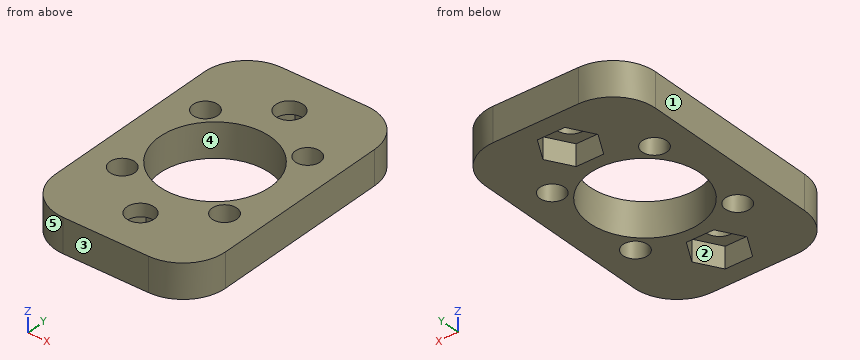
```python
from build123d import *

# Parameters (mm, degrees)
SKETCH_W     = 20
SKETCH_H     = 31.5
SKETCH_R     = 1.6
SKETCH_R_2   = 6.5
SKETCH_R_3   = 1.45
PAD_DEPTH    = 4
POCKET_DEPTH = 2.5
FILLET_R     = 5


with BuildPart() as part:
    # Sketch → Pad (new body)
    with BuildSketch(Plane.XY):
        Rectangle(SKETCH_W, SKETCH_H)
        with Locations((0, 10.75)):
            Circle(SKETCH_R, mode=Mode.SUBTRACT)
        with Locations((0, -10.75)):
            Circle(SKETCH_R, mode=Mode.SUBTRACT)
        Circle(SKETCH_R_2, mode=Mode.SUBTRACT)
        with Locations((6, 6)):
            Circle(SKETCH_R_3, mode=Mode.SUBTRACT)
        with Locations((6, -6)):
            Circle(SKETCH_R_3, mode=Mode.SUBTRACT)
        with Locations((-6, -6)):
            Circle(SKETCH_R_3, mode=Mode.SUBTRACT)
        with Locations((-6, 6)):
            Circle(SKETCH_R_3, mode=Mode.SUBTRACT)
    extrude(amount=PAD_DEPTH)

    # Sketch001 → Pocket (cut)
    with BuildSketch(Plane.XY):
        Polygon((-1.616581, 7.95), (1.616581, 7.95), (3.233162, 10.75), (1.616581, 13.55), (-1.616581, 13.55), (-3.233162, 10.75), align=None)
        Polygon((-1.616581, -7.95), (-3.233162, -10.75), (-1.616581, -13.55), (1.616581, -13.55), (3.233162, -10.75), (1.616581, -7.95), align=None)
    extrude(amount=POCKET_DEPTH, mode=Mode.SUBTRACT)

    # Fillet
    fillet_edges = [part.edges().sort_by_distance(p)[0] for p in [
        (10, -15.75, 2),
        (10, 15.75, 2),
        (-10, 15.75, 2),
        (-10, -15.75, 2),
    ]]
    fillet(fillet_edges, radius=FILLET_R)


solid = part.part
```
Could you check a few things on this model? Use its own coordinates, in mm. Face numbers are marked on the shaded views. A direction names the side the tool comes from. Round coordinates to 2 decimals unless told otherwise and drop trailing zeros. Loops run counter-clockwise (first coordinate to the right, second up) from the corner with the lowest first, then second, coordinate; pieces in that order, holes last. Notation, with made-up numbers: (-35.75, -15) - (21.25, -15) arc R22 cw to (21.25, 9) - close; hole circle Ø7 at (49, 9). An arc over 180 degrees is marked (long way). Answer in a Markdown table with one row per item. Add a question column.
(1) I need wall thicknesses on line 1 along Y through (x, z) = (0, 2.2); line 2 along Y through (x, z) = (0, 3.75); line 3 along X through (y, z) = (-10.75, 3.55). Which ranges of each line are inside material? Lowest first, please.
(2) If we section it at D-D (y = 0): Please give me the cut outline in (x, z).
(3) For the marked faces 1 and 2, which set-ups out of +Z, -Z, +X, -X, +Y, -Y let a thin tool reach every point of the face, with its end or its side?
(4) I'm going to push a flat-ended pin straight in: pin 1 (10 mm diameter, centred on x = 1.5, y = 2.5, fed in from +Z). Where does the tip first touch, or does it pass through?
(5) If we mould it in two halves opening along X, with no side actions, what happens to the marked faces 3, 4 and 5? For each: pulls with the +X half, pulls with the -X half, needs draft (parallel to the pull), parting line crosses it, or undercut.
(6) If we section it at A-A (y = -6): Please give me the cut outline in (x, z).
(7) If we section it at C-C (x = 6): Please give me the cut outline in (y, z), plus the area to 3 significant figures.
(8) If we section it at B-B (z = 0.7): Please give me the cut outline in (x, y).
Model answer:
| question | item | result |
|---|---|---|
| 1 | line 1 | y = -15.75 to -13.55, -7.95 to -6.5, 6.5 to 7.95, 13.55 to 15.75 |
| 1 | line 2 | y = -15.75 to -12.35, -9.15 to -6.5, 6.5 to 9.15, 12.35 to 15.75 |
| 1 | line 3 | x = -10 to -1.6, 1.6 to 10 |
| 2 | outline | (-10, 0) - (-6.5, 0) - (-6.5, 4) - (-10, 4) - close; (6.5, 0) - (10, 0) - (10, 4) - (6.5, 4) - close |
| 3 | face 1 | +Z, -Z, -X, +Y, -Y |
| 3 | face 2 | -Z |
| 4 | pin 1 | stops at z = 4 |
| 5 | face 3 | needs draft |
| 5 | face 4 | undercut |
| 5 | face 5 | pulls with the -X half |
| 6 | outline | (-10, 0) - (-7.45, 0) - (-7.45, 4) - (-10, 4) - close; (-4.55, 0) - (-2.5, 0) - (-2.5, 4) - (-4.55, 4) - close; (2.5, 0) - (4.55, 0) - (4.55, 4) - (2.5, 4) - close; (7.45, 0) - (10, 0) - (10, 4) - (7.45, 4) - close |
| 7 | outline | (-15.65, 0) - (-7.45, 0) - (-7.45, 4) - (-15.65, 4) - close; (-4.55, 0) - (-2.5, 0) - (-2.5, 4) - (-4.55, 4) - close; (2.5, 0) - (4.55, 0) - (4.55, 4) - (2.5, 4) - close; (7.45, 0) - (15.65, 0) - (15.65, 4) - (7.45, 4) - close |
| 7 | area | 82.0 mm² |
| 8 | outline | (-10, -10.75) arc R5 ccw to (-5, -15.75) - (5, -15.75) arc R5 ccw to (10, -10.75) - (10, 10.75) arc R5 ccw to (5, 15.75) - (-5, 15.75) arc R5 ccw to (-10, 10.75) - close; hole circle Ø2.9 at (-6, -6); hole circle Ø2.9 at (-6, 6); hole circle Ø13 at (0, 0); hole (-3.23, -10.75) - (-1.62, -13.55) - (1.62, -13.55) - (3.23, -10.75) - (1.62, -7.95) - (-1.62, -7.95) - close; hole (-3.23, 10.75) - (-1.62, 7.95) - (1.62, 7.95) - (3.23, 10.75) - (1.62, 13.55) - (-1.62, 13.55) - close; hole circle Ø2.9 at (6, -6); hole circle Ø2.9 at (6, 6) |
